Read the model definition and answer for the solid it produces. Units are mm, in the model's axes. A direction names the side the tool comes from. Round coordinates to 2 decimals unless told otherwise and drop trailing zeros. Write each loop counter-clockwise with the first axis right and the second up, starting at its lowest first coordinate (ties: lowest second). Pieces come first, ordered by that corner, then holes. Notation, with made-up numbers: (61.25, -23) - (96.25, -23) arc R30 ccw to (96.25, 4) - close; hole circle Ø5 at (-4.75, 68.25). An arc over 180 degrees is marked (long way). One line per item, written item: value. Start each with the question number.
(1) For faces 1 (the face through (0, -18, 28)), 2 (the face through (-24, 0, 29)), determine the directions among +Z, -Z, +X, -X, +Y, -Y from which every point of the face is accessible in a straight line to the end or side of a thin tool.
(2) A cutting plane is placed at A-A, the plane z = 42.5. Determine the outline of the cut face in (x, y).
(3) Flat-ended cylindrical pins translate along their axes: pin 1 Ø5 at (x, y) = (20, 8) entering from +Z; pin 2 Ø1.5 at (x, y) = (0.5, 15) entering from +Z. Find the tip coordinate at first contact, or state that the pin passes through.
(4) Find the intervals of material crossed by L1, parallel to Y at x = 17, z = 13.5; L2, parallel to X at y = 10.5, z = 45; L3, parallel to Z at x = -18.5, y = -11, in increasing order.
(5) The mould has two halves that part along X. Classify faces 3 (the face through (0, 5, 0)), 4 (the face through (26.57, -17.55, 28.65)), 5 (the face through (24, 0, 29)): +X half, -X half, draft (parallel to the pull), parting line (faces both ways), or undercut.
from build123d import *

# Parameters (mm, degrees)
F0_W     = 54
F0_H     = 36
F1_DEPTH = 58
F2_T     = -3
F3_W     = 54
F3_H     = 58
F4_DEPTH = 10
F5_R     = 1.49999


# Not quite as in the source:
# - a fillet or chamfer is up to 0.001 mm smaller than in the source, because OpenCascade refuses the exact size


with BuildPart() as f1:
    # F0 (on Top) → F1 (new body)
    with BuildSketch(Plane.XY):
        Rectangle(F0_W, F0_H)
    extrude(amount=F1_DEPTH)

    # F2
    f2_openings = [f1.faces().sort_by_distance(p)[0] for p in [
        (0, 0, 58),
    ]]
    offset(amount=F2_T, openings=f2_openings)

    # F3 (on face) → F4 (join)
    with BuildSketch(Plane(origin=(0, 18, 0), x_dir=(-1, 0, 0), z_dir=(0, 1, 0))):
        with Locations((0, 29)):
            Rectangle(F3_W, F3_H)
    extrude(amount=F4_DEPTH)

    # F5 (radius 1.5 in the source; OpenCascade refuses exactly that, so slightly less here)
    f5_edges = [f1.edges().sort_by_distance(p)[0] for p in [
        (0, -18, 58),
        (27, 5, 58),
        (0, 28, 58),
        (-27, 5, 58),
        (0, -15, 58),
        (-24, 0, 58),
        (0, 15, 58),
        (24, 0, 58),
        (-27, -18, 29),
        (27, -18, 29),
    ]]
    fillet(f5_edges, radius=F5_R)


solid = f1.part
Here are the results:
1. face 1: +Z, -Z, +X, -X, -Y
1. face 2: +Z
2. outline: (-27, -16.5) arc R1.5 ccw to (-25.5, -18) - (25.5, -18) arc R1.5 ccw to (27, -16.5) - (27, 28) - (-27, 28) - close; hole (-24, -15) - (24, -15) - (24, 15) - (-24, 15) - close
3. pin 1: z = 3
3. pin 2: z = 57.8
4. L1: -18 to -15, 15 to 28
4. L2: -27 to -24, 24 to 27
4. L3: 0 to 3
5. face 3: draft
5. face 4: +X half
5. face 5: undercut
